from build123d import *

# Parameters (mm, degrees)
SKETCH1_W           = 65
SKETCH1_H           = 45
BOSS_EXTRUDE1_DEPTH = 1
SKETCH2_W           = 10
SKETCH2_H           = 40.24
BOSS_EXTRUDE2_DEPTH = 27.06
CUT_EXTRUDE1_START  = -10
SKETCH3_R           = 0.9
CUT_EXTRUDE1_DEPTH  = 59.475391695
CUT_EXTRUDE2_REACH  = 74.435
SKETCH4_W           = 8.1
SKETCH4_H           = 7.5
SKETCH5_W           = 40.75
SKETCH5_H           = 10
BOSS_EXTRUDE3_DEPTH = 27.06
SKETCH6_W           = 16.07
SKETCH6_H           = 7.5
CUT_EXTRUDE3_DEPTH  = 50.75
SKETCH7_W           = 40.75
SKETCH7_H           = 10
CUT_EXTRUDE4_DEPTH  = 27.06


with BuildPart() as part:
    # Sketch1 → Boss-Extrude1 (new body)
    with BuildSketch(Plane(origin=(0, 0, 0), x_dir=(1, 0, 0), z_dir=(0, 1, 0))):
        Rectangle(SKETCH1_W, SKETCH1_H)
    extrude(amount=BOSS_EXTRUDE1_DEPTH)

    # Sketch2 → Boss-Extrude2 (add)
    with BuildSketch(Plane(origin=(0, 1, 0), x_dir=(1, 0, 0), z_dir=(0, 1, 0))):
        with Locations((25.375, 0)):
            Rectangle(SKETCH2_W, SKETCH2_H)
    boss_extrude2 = extrude(amount=BOSS_EXTRUDE2_DEPTH)

    # Sketch3 → Cut-Extrude1 (cut)
    with BuildSketch(Plane(origin=(0, 28.06, 0), x_dir=(1, 0, 0), z_dir=(0, 1, 0)).offset(CUT_EXTRUDE1_START)):
        with Locations(Location((24.175, 5.45, 0), (0, 0, 90))):
            Circle(SKETCH3_R)
        with Locations(Location((24.175, -4.25, 0), (0, 0, 90))):
            Circle(SKETCH3_R)
    cut_extrude1 = extrude(amount=CUT_EXTRUDE1_DEPTH, mode=Mode.SUBTRACT)

    # Mirror3: Boss-Extrude2, Cut-Extrude1 across plane
    add(boss_extrude2.mirror(Plane(origin=(0, 0, 0), x_dir=(0, 0, 1), z_dir=(1, 0, 0))))
    add(cut_extrude1.mirror(Plane(origin=(0, 0, 0), x_dir=(0, 0, 1), z_dir=(1, 0, 0))), mode=Mode.SUBTRACT)

    # Sketch4 → Cut-Extrude2 (cut, up to next)
    with BuildSketch(Plane.ZY.offset(30.375), mode=Mode.PRIVATE) as cut_extrude2_sk1:
        with Locations((0, 4.75)):
            Rectangle(SKETCH4_W, SKETCH4_H)
    cut_extrude2_tool1 = extrude(cut_extrude2_sk1.sketch, amount=-CUT_EXTRUDE2_REACH, mode=Mode.PRIVATE) & part.part
    add(cut_extrude2_tool1.solids().sort_by_distance((-30.375, 4.75, 0))[0], mode=Mode.SUBTRACT)

    # Sketch5 → Boss-Extrude3 (add)
    with BuildSketch(Plane(origin=(0, 1, 0), x_dir=(1, 0, 0), z_dir=(0, 1, 0))):
        with Locations((0, 15.12)):
            Rectangle(SKETCH5_W, SKETCH5_H)
    boss_extrude3 = extrude(amount=BOSS_EXTRUDE3_DEPTH)

    # Mirror4: Boss-Extrude3 across plane
    add(boss_extrude3.mirror(Plane.XY))

    # Sketch6 → Cut-Extrude3 (cut)
    with BuildSketch(Plane.ZY.offset(30.375)):
        with Locations((-12.085, 4.75)):
            Rectangle(SKETCH6_W, SKETCH6_H)
    extrude(amount=-CUT_EXTRUDE3_DEPTH, mode=Mode.SUBTRACT)

    # Sketch7 → Cut-Extrude4 (cut)
    with BuildSketch(Plane(origin=(0, 28.06, 0), x_dir=(1, 0, 0), z_dir=(0, 1, 0))):
        with Locations((0, 15.12)):
            Rectangle(SKETCH7_W, SKETCH7_H)
    extrude(amount=-CUT_EXTRUDE4_DEPTH, mode=Mode.SUBTRACT)


solid = part.part
Input: part model. Units: mm. Frame: model coordinates. A direction names the side the tool comes from. Give positions to 0.01 mm unless a question says otherwise; leave off trailing zeros. Loops run counter-clockwise (first coordinate to the right, second up) from the corner with the lowest first, then second, coordinate; pieces in that order, holes last. Notation, with made-up numbers: (8.25, -30.75) - (13.25, -30.75) arc R10 cw to (13.25, -12.75) - close; hole circle Ø7 at (46, 21.25). An arc over 180 degrees is marked (long way). Use CSV: the item, a comma, the result in double quotes. Start each with the question number.
Item 1: Contact query for flat-ended pins moving along their axis: P1, Ø4, axis at x = -27.5, y = 5, coming from the -Z side; P2, Ø3, axis at x = -23, y = 21, coming from the -Z side; P3, Ø8, axis at y = 21.5, z = -5, coming from the +X side (3 decimals); P4, Ø10, axis at y = 5, z = -15.5, coming from the +X side. Output: stop coordinate, or through.
Item 2: Mould query, pull axis Y, two halves, no side actions, for faces 4 (the flat face through (-25, 8.5, -8)), 5 (the flat face through (-25, 5, 4.05)), 6 (the flat face through (-24, 18.06, 4)), 7 (the flat face through (20.375, 14, -5)). Classes: pulls with the +Y half, pulls with the -Y half, needs draft (parallel to the pull), parting line crosses it, or undercut.
Item 3: Reachability of faces 1 (the flat face through (-30.375, 17, 0)), 2 (the flat face through (0, 14, 10.12)), 3 (the cylindrical face through (-25.054, 22.99, -5.255)) from +Z, -Z, +X, -X, +Y, -Y: full face, straight path, thin tool, end or side. Return the list, or none.
Item 4: Section D-D on y = 22.75. Return loops of the section in (x, z) (3 decimals), then the cut area to 3 significant figures.
Item 5: Section C-C on x = 10. Return loops of the section in (y, z), then the cut area to 3 significant figures.
Item 6: Section A-A on z = -11.5. Return loops of the section in (x, y) (3 decimals), then the cut area to 3 significant figures.
Item 7: Line query: line 1 (X direction, y = 21, z = 4.25) (3 decimals); line 2 (X direction, y = 24.5, z = -0.5) (3 decimals); line 3 (Y direction, x = 4, z = 9). Output: solid intervals per line, ascending.
Item 8: Section B-B on z = -5.45. Return loops of the section in (x, y) (3 decimals), then the cut area to 3 significant figures.
Ans:
1,P1,"stops at z = 4.05"
1,P2,"stops at z = -20.12"
1,P3,"stops at x = 30.375"
1,P4,"stops at x = 32.5"
2,face 4,"undercut"
2,face 5,"undercut"
2,face 6,"pulls with the +Y half"
2,face 7,"needs draft"
3,face 1,"+Z, -Z, -X, +Y"
3,face 2,"-Z, +Y"
3,face 3,"+Y"
4,outline,"(-30.375, -20.12) - (-20.375, -20.12) - (-20.375, 10.12) - (20.375, 10.12) - (20.375, -20.12) - (30.375, -20.12) - (30.375, 20.12) - (-30.375, 20.12) - close; hole circle Ø1.8 at (-24.175, -5.45); hole circle Ø1.8 at (-24.175, 4.25); hole circle Ø1.8 at (24.175, -5.45); hole circle Ø1.8 at (24.175, 4.25)"
4,area,"1,200 mm2"
5,outline,"(0, -22.5) - (1, -22.5) - (1, 10.12) - (28.06, 10.12) - (28.06, 20.12) - (1, 20.12) - (1, 22.5) - (0, 22.5) - close"
5,area,"316 mm2"
6,outline,"(-32.5, 0) - (32.5, 0) - (32.5, 1) - (30.375, 1) - (30.375, 28.06) - (20.375, 28.06) - (20.375, 1) - (-32.5, 1) - close; (-30.375, 8.5) - (-20.375, 8.5) - (-20.375, 28.06) - (-30.375, 28.06) - close"
6,area,"531 mm2"
7,line 1,"x = -30.375 to -25.075, -23.275 to -20.375, 20.375 to 23.275, 25.075 to 30.375"
7,line 2,"x = -30.375 to -20.375, 20.375 to 30.375"
7,line 3,"y = 0 to 1"
8,outline,"(-32.5, 0) - (32.5, 0) - (32.5, 1) - (30.375, 1) - (30.375, 28.06) - (25.075, 28.06) - (25.075, 18.06) - (23.275, 18.06) - (23.275, 28.06) - (20.375, 28.06) - (20.375, 1) - (-32.5, 1) - close; (-30.375, 8.5) - (-20.375, 8.5) - (-20.375, 28.06) - (-23.275, 28.06) - (-23.275, 18.06) - (-25.075, 18.06) - (-25.075, 28.06) - (-30.375, 28.06) - close"
8,area,"495 mm2"
